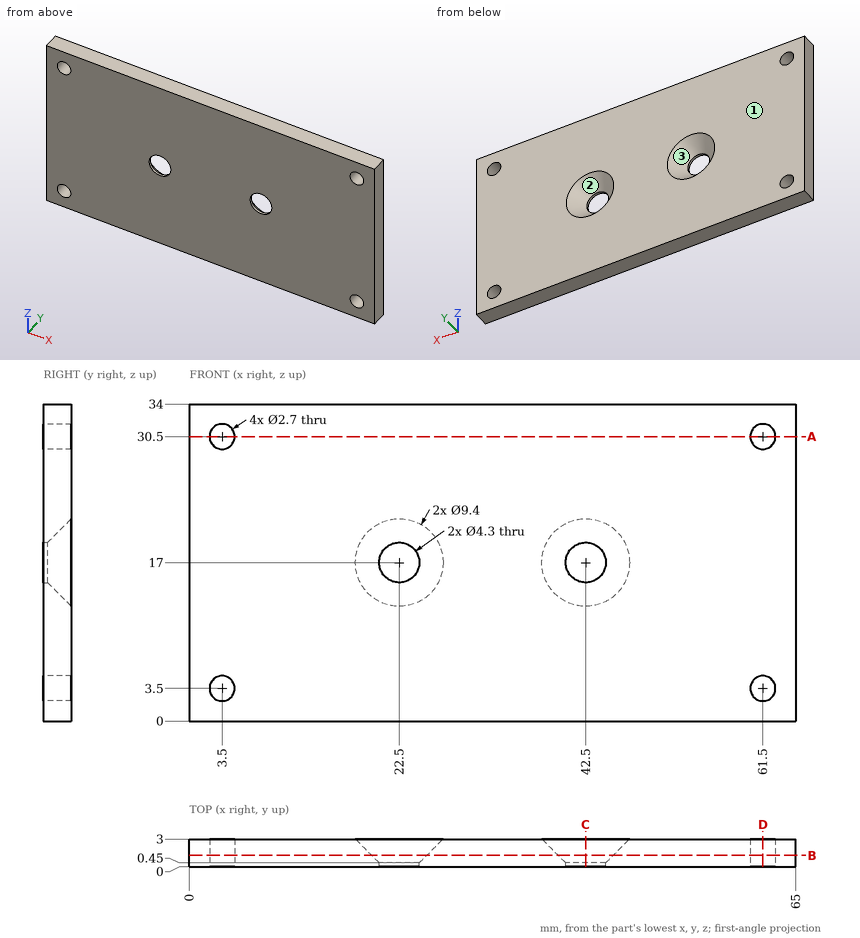
Study the drawing (mm; zero at the part's minimum x, y, z) and answer. Give positions to 0.01 mm unless a question says otherwise; leave off trailing zeros. Order: outer loops, then holes, each group sorted by start corner. A loop starts at its lowest first (then second) coordinate and runs counter-clockwise, first axis right, second up.
1) Find section A-A on z = 30.5. Write down the section's boundary in (x, y), then the cut area to 3 significant figures.
Reported:
outline: (0, 0) - (2.15, 0) - (2.15, 3) - (0, 3) - close; (4.85, 0) - (60.15, 0) - (60.15, 3) - (4.85, 3) - close; (62.85, 0) - (65, 0) - (65, 3) - (62.85, 3) - close
area: 179 mm2
2) Consider line 1 along Z through (x, y) = (3.5, 1.4); line 2 along X through (y, z) = (0.8, 30.5); line 3 along Z through (x, y) = (22.5, 0.15). Determine where each line is inside the solid, lowest interval first.
Reported:
line 1: z = 0 to 2.15, 4.85 to 29.15, 31.85 to 34
line 2: x = 0 to 2.15, 4.85 to 60.15, 62.85 to 65
line 3: z = 0 to 14.85, 19.15 to 34
3) Determine the mould class of the marked faces 1, 2 and 3 for opening direction Z: pulls with the +Z half, pulls with the -Z half, needs draft (parallel to the pull), parting line crosses it, or undercut.
Reported:
face 1: needs draft
face 2: undercut
face 3: undercut
4) Find section C-C on x = 42.5. Write down the section's boundary in (y, z).
Reported:
outline: (0, 0) - (3, 0) - (3, 12.3) - (0.45, 14.85) - (0, 14.85) - close; (0, 19.15) - (0.45, 19.15) - (3, 21.7) - (3, 34) - (0, 34) - close
5) Find section B-B on y = 1.25. Write down the section's boundary in (x, z).
Reported:
outline: (0, 0) - (65, 0) - (65, 34) - (0, 34) - close; hole circle Ø2.7 at (3.5, 3.5); hole circle Ø2.7 at (3.5, 30.5); hole circle Ø5.9 at (22.5, 17); hole circle Ø5.9 at (42.5, 17); hole circle Ø2.7 at (61.5, 3.5); hole circle Ø2.7 at (61.5, 30.5)
6) Given P1, Ø7, axis at x = 22.5, z = 17, coming from the -Y side; P2, Ø2, axis at x = 3.5, z = 3.5, coming from the -Y side; P3, Ø7, axis at x = 42.5, z = 17, coming from the +Y side, each flat-ended and moving along its own axis, determine where each tip first touches the part or whether it passes through.
Reported:
P1: stops at y = 0
P2: passes through
P3: stops at y = 1.8
7) Find section D-D on x = 61.5. Write down the section's boundary in (y, z), then the cut area to 3 significant figures.
Reported:
outline: (0, 0) - (3, 0) - (3, 2.15) - (0, 2.15) - close; (0, 4.85) - (3, 4.85) - (3, 29.15) - (0, 29.15) - close; (0, 31.85) - (3, 31.85) - (3, 34) - (0, 34) - close
area: 85.8 mm2
